Source: CAD feature listing. Evaluate the final solid. Frame: model axes, mm. A direction names the side the tool comes from. Coordinates: 2 decimals unless noted, no trailing zeros. Order: outer loops, then holes, each group sorted by start corner. A loop starts at its lowest first (then second) coordinate and runs counter-clockwise, first axis right, second up.
Autodesk Inventor part; units mm, degrees
ref_plane "YZ Plane" through (0, 0, 0) normal (1, 0, 0) x (0, 1, 0)
ref_plane "XZ Plane" through (0, 0, 0) normal (0, 1, 0) x (-1, 0, 0)
ref_plane "XY Plane" through (0, 0, 0) normal (0, 0, 1) x (1, 0, 0)
sketch "Sketch1" plane through (0, 0, 0) normal (0, 1, 0) x (-1, 0, 0)
  line L0 (0, 0) -> (42, 0)
  line L1 (42, 0) -> (42, -73)
  line L2 (42, -73) -> (0, -73)
  line L3 (0, -73) -> (0, 0)
  dimension "d0" = 42
  dimension "d1" = 73
extrude "Extrusion1" add sketch "Sketch1" along normal blind 10
hole "Hole1" at (-37, 10, -5) direction (0, -1, 0) diameter 4.4 end through all
hole "Hole2" at (-37, 10, -68) direction (0, -1, 0) diameter 4.4 end through all
hole "Hole3" at (-5, 10, -68) direction (0, -1, 0) diameter 4.4 end through all
hole "Hole4" at (-5, 10, -5) direction (0, -1, 0) diameter 4.4 end through all
sketch "Sketch2" plane through (0, 0, 0) normal (1, 0, 0) x (0, 0, -1)
  line L0 (10, 10) -> (63, 10)
  line L1 (63, 10) -> (63, 0)
  line L2 (63, 0) -> (10, 0)
  line L3 (10, 0) -> (10, 10)
  line L4 (0, 10) -> (73, 10)
  line L5 (73, 0) -> (0, 0)
  dimension "d40" = 10
  dimension "d41" = 10
extrude "Extrusion2" add sketch "Sketch2" along normal blind 10
sketch "Sketch4" plane through (-42, 0, -73) normal (-1, 0, 0) x (0, 0, 1)
  line L0 (10, 10) -> (63, 10)
  line L1 (63, 10) -> (63, 0)
  line L2 (63, 0) -> (10, 0)
  line L3 (10, 0) -> (10, 10)
  line L4 (73, 0) -> (0, 0)
  line L5 (0, 10) -> (73, 10)
  dimension "d44" = 10
  dimension "d45" = 10
extrude "Extrusion3" add sketch "Sketch4" along normal blind 10
sketch "Sketch5" plane through (0, 10, 0) normal (0, 1, 0) x (1, 0, 0)
  line L0 (-42, 53) -> (0, 53)
  line L1 (0, 53) -> (0, 20)
  line L2 (0, 20) -> (-42, 20)
  line L3 (-42, 20) -> (-42, 53)
  line L4 (10, 63) -> (10, 10)
  line L5 (0, 73) -> (-42, 73)
  line L6 (-52, 10) -> (-52, 63)
  point P0 (0, 0)
  dimension "d48" = 10
  dimension "d49" = 20
  dimension "d50" = 20
  dimension "d51" = 10
extrude "Extrusion4" cut sketch "Sketch5" against normal up to next
sketch "Sketch6" plane through (0, 10, 0) normal (0, 1, 0) x (1, 0, 0)
  line L0 (-32, 63) -> (-10, 63)
  line L1 (-10, 63) -> (-10, 53)
  line L2 (-10, 53) -> (-32, 53)
  line L3 (-32, 53) -> (-32, 63)
  line L4 (-32, 20) -> (-10, 20)
  line L5 (-10, 20) -> (-10, 10)
  line L6 (-10, 10) -> (-32, 10)
  line L7 (-32, 10) -> (-32, 20)
  line L8 (-42, 53) -> (0, 53)
  line L9 (0, 20) -> (-42, 20)
  line L10 (0, 63) -> (0, 73)
  line L11 (-42, 73) -> (-42, 63)
  line L12 (0, 0) -> (0, 10)
  line L13 (-42, 10) -> (-42, 0)
  line L14 (-42, 63) -> (-52, 63)
  line L15 (0, 10) -> (10, 10)
  dimension "d54" = 10
  dimension "d55" = 10
  dimension "d56" = 10
  dimension "d57" = 10
extrude "Extrusion5" cut sketch "Sketch6" against normal up to next
properties part number "bottomplate"
1. Section query C-C on x = -13.5. Return loops of the section in (y, z).
Findings:
outline: (0, -73) - (10, -73) - (10, -63) - (0, -63) - close; (0, -10) - (10, -10) - (10, 0) - (0, 0) - close
2. Pin query (flat end, axial travel): P1, Ø4, axis at x = -5, z = -5, coming from the -Y side; P2, Ø3, axis at y = 7, z = -6, coming from the -X side; P3, Ø5, axis at x = 5.5, y = 4.5, coming from the -Z side. Return the tip coordinate at first contact, or that it passes through.
Findings:
P1: passes through
P2: stops at x = -42
P3: stops at z = -63
3. Access query for faces 1 (the face through (-47, 5, -63)), 2 (the face through (-42, 5, -5)), 3 (the face through (0, 5, -37)). Directions: +Z, -Z, +X, -X, +Y, -Y. A direction counts if a zero-diameter tool reaches every point of the face in a straight line with its end or side. Return the directions, or none.
Findings:
face 1: -Z, -X, +Y, -Y
face 2: +Z, -X, +Y, -Y
face 3: +Y, -Y
4. Section query A-A on x = -5. Return loops of the section in (y, z), plus the area to 3 significant figures.
Findings:
outline: (0, -73) - (10, -73) - (10, -70.2) - (0, -70.2) - close; (0, -65.8) - (10, -65.8) - (10, -53) - (0, -53) - close; (0, -20) - (10, -20) - (10, -7.2) - (0, -7.2) - close; (0, -2.8) - (10, -2.8) - (10, 0) - (0, 0) - close
area: 312 mm2
5. Ray query, line 1 (X direction, y = 6.25, z = -68); line 2 (Z direction, x = -5, y = 2); line 3 (Z direction, x = -26.5, y = 4.5). Return the intervals inside material, ascending.
Findings:
line 1: x = -42 to -39.2, -34.8 to -7.2, -2.8 to 0
line 2: z = -73 to -70.2, -65.8 to -53, -20 to -7.2, -2.8 to 0
line 3: z = -73 to -63, -10 to 0
6. Section query B-B on z = -68. Return loops of the section in (x, y).
Findings:
outline: (-42, 0) - (-39.2, 0) - (-39.2, 10) - (-42, 10) - close; (-34.8, 0) - (-7.2, 0) - (-7.2, 10) - (-34.8, 10) - close; (-2.8, 0) - (0, 0) - (0, 10) - (-2.8, 10) - close
7. Section query D-D on z = -56. Return loops of the section in (x, y), plus the area to 3 significant figures.
Findings:
outline: (-52, 0) - (-32, 0) - (-32, 10) - (-52, 10) - close; (-10, 0) - (10, 0) - (10, 10) - (-10, 10) - close
area: 400 mm2
8. Draft query along Z for faces 4 (the face through (-47, 5, -10)), 5 (the face through (-6.8, 10, -19.8)), 6 (the face through (-21, 5, -63)). Return one class per face: released by +Z, released by -Z, zero draft, split by the parting line, or undercut.
Findings:
face 4: released by +Z
face 5: zero draft
face 6: undercut
